Work out the finished part from the listing and answer in its coordinate system (mm). A direction names the side the tool comes from. Give positions to 0.01 mm unless a question says otherwise; leave off trailing zeros. Loops run counter-clockwise (first coordinate to the right, second up) from the corner with the lowest first, then second, coordinate; pieces in that order, holes last. Notation, with made-up numbers: M 48.25,9 L 58.25,9 A28 cw 58.25,38 Z; hole C -36,-32 d8. An arc over 180 degrees is marked long. Write item = value, one per line. Start each with the question number.
1. The mould has two halves that part along X. Classify faces 1 (the face through (-1.93, 1.97, -2.52)), 2 (the face through (6, 2, 7.175)), 3 (the face through (-5.103, 1.972, 5.044)): released by +X, released by -X, zero draft, split by the parting line, or undercut.
2. Consider L1, parallel to X at y = 1.6, z = 0 (3 decimals); L2, parallel to Z at x = 6.25, y = 0.3 (3 decimals); L3, parallel to X at y = 2.75, z = -0.75 (3 decimals). Determine where each line is inside the solid, lowest interval first. Write a range as [from, to].
3. Flat-ended cylindrical pins translate along their axes: pin 1 Ø1 at (x, y) = (18, 0.5) entering from +Z; pin 2 Ø1.5 at (x, y) = (0.5, 1.5) entering from +Z (3 decimals). Find the tip coordinate at first contact, or state that the pin passes through.
4. For faces 4 (the face through (6, 2, -7.175)), 5 (the face through (17.701, 1.972, 9.215)), determine the directions among +Z, -Z, +X, -X, +Y, -Y from which every point of the face is accessible in a straight line to the end or side of a thin tool.
5. Section C-C on y = 2.1 is taken. Determine the outline of the cut face in (x, z) (3 decimals).
6. Section A-A on x = 0 is taken. Determine the outline of the cut face in (y, z) (3 decimals), plus the area to 3 significant figures.
7. Section B-B on z = 0 is taken. Determine the outline of the cut face in (x, y) (3 decimals).
```python
from build123d import *

# Parameters (mm, degrees)
SKETCH1_R           = 3.175
BOSS_EXTRUDE1_DEPTH = 4


with BuildPart() as part:
    # Sketch1 → Boss-Extrude1 (new body)
    with BuildSketch(Plane(origin=(0, 0, 0), x_dir=(1, 0, 0), z_dir=(0, 1, 0))):
        Polygon((-7.175, 2.97198231), (-7.175, -2.97198231), (-2.97198231, -7.175), (15.660281374, -7.175), (19.798989873, -11.313708499), (22.627416998, -8.485281374), (22.627416998, 8.485281374), (19.798989873, 11.313708499), (15.660281374, 7.175), (-2.97198231, 7.175), align=None)
        with Locations(Location((0, 0, 0), (0, 0, 270))):
            Circle(SKETCH1_R, mode=Mode.SUBTRACT)
    extrude(amount=BOSS_EXTRUDE1_DEPTH)


solid = part.part
```
Verdict:
q1.face_1 = undercut
q1.face_2 = zero draft
q1.face_3 = released by -X
q2.L1 = [-7.175, -3.175], [3.175, 22.627]
q2.L2 = [-7.175, 7.175]
q2.L3 = [-7.175, -3.085], [3.085, 22.627]
q3.pin_1 = 10.01
q3.pin_2 = 7.175
q4.face_4 = -Z, -X, +Y, -Y
q4.face_5 = +Z, -X, +Y, -Y
q5.outline = M -7.175,-2.972 L -2.972,-7.175 L 15.66,-7.175 L 19.799,-11.314 L 22.627,-8.485 L 22.627,8.485 L 19.799,11.314 L 15.66,7.175 L -2.972,7.175 L -7.175,2.972 Z; hole C 0,0 d6.35
q6.outline = M 0,-7.175 L 4,-7.175 L 4,-3.175 L 0,-3.175 Z; M 0,3.175 L 4,3.175 L 4,7.175 L 0,7.175 Z
q6.area = 32.0 mm2
q7.outline = M -7.175,0 L -3.175,0 L -3.175,4 L -7.175,4 Z; M 3.175,0 L 22.627,0 L 22.627,4 L 3.175,4 Z
